Part model, mm, in its own coordinate system. Round coordinates to 2 decimals unless told otherwise and drop trailing zeros. Loops run counter-clockwise (first coordinate to the right, second up) from the corner with the lowest first, then second, coordinate; pieces in that order, holes last.
from build123d import *

# Parameters (mm, degrees)
SKETCH1_R                = 6
BOSS_EXTRUDE1_DEPTH      = 254
BOSS_EXTRUDE1_DEPTH_BACK = 56
CUT_EXTRUDE3_START       = -56
SKETCH2_W                = 4
SKETCH2_H                = 5
CUT_EXTRUDE3_DEPTH       = 20
CUT_EXTRUDE3_DEPTH_BACK  = 0.0001
CUT_EXTRUDE4_START       = 254
SKETCH2_2_W              = 4
SKETCH2_2_H              = 5
CUT_EXTRUDE4_DEPTH       = 50
CUT_EXTRUDE6_START       = -56
SKETCH3_W                = 4
SKETCH3_H                = 10
CUT_EXTRUDE6_DEPTH       = 6


with BuildPart() as part:
    # Sketch1 → Boss-Extrude1 (new body, two sides)
    with BuildSketch(Plane(origin=(0, 0, 0), x_dir=(1, 0, 0), z_dir=(0, 1, 0))) as boss_extrude1_sk:
        Circle(SKETCH1_R)
    extrude(amount=BOSS_EXTRUDE1_DEPTH)
    extrude(boss_extrude1_sk.sketch, amount=-BOSS_EXTRUDE1_DEPTH_BACK)

    # Sketch2 → Cut-Extrude3 (cut, two sides)
    with BuildSketch(Plane(origin=(0, 0, 0), x_dir=(1, 0, 0), z_dir=(0, 1, 0)).offset(CUT_EXTRUDE3_START)) as cut_extrude3_sk:
        with Locations((0, -6)):
            Rectangle(SKETCH2_W, SKETCH2_H)
    extrude(amount=CUT_EXTRUDE3_DEPTH, mode=Mode.SUBTRACT)
    extrude(cut_extrude3_sk.sketch, amount=-CUT_EXTRUDE3_DEPTH_BACK, mode=Mode.SUBTRACT)

    # Sketch2<2> → Cut-Extrude4 (cut)
    with BuildSketch(Plane(origin=(0, 0, 0), x_dir=(1, 0, 0), z_dir=(0, 1, 0)).offset(CUT_EXTRUDE4_START)):
        with Locations((0, -6)):
            Rectangle(SKETCH2_2_W, SKETCH2_2_H)
    extrude(amount=-CUT_EXTRUDE4_DEPTH, mode=Mode.SUBTRACT)

    # Sketch3 → Cut-Extrude6 (cut)
    with BuildSketch(Plane(origin=(0, 0, 0), x_dir=(1, 0, 0), z_dir=(0, 1, 0)).offset(CUT_EXTRUDE6_START)):
        with Locations((0, -6)):
            Rectangle(SKETCH3_W, SKETCH3_H)
    extrude(amount=CUT_EXTRUDE6_DEPTH, mode=Mode.SUBTRACT)


solid = part.part
1) Slice it at A-A, the plane x = 0. Give the cut face in (y, z), then the cut area to 3 significant figures.
Values:
outline: (-56, -6) - (254, -6) - (254, 3.5) - (204, 3.5) - (204, 6) - (-36, 6) - (-36, 3.5) - (-50, 3.5) - (-50, 1) - (-56, 1) - close
area: 3,530 mm2
2) Slice it at B-B, the plane y = 12.5. Give the cut face in (x, z).
Values:
outline: circle Ø12 at (0, 0)
3) Slice it at C-C, the plane z = -2. Give the cut face in (x, y), then the cut area to 3 significant figures.
Values:
outline: (-5.66, -56) - (5.66, -56) - (5.66, 254) - (-5.66, 254) - close
area: 3,510 mm2
4) Wall check: line 1 along X through (y, z) = (216.5, -0.75); line 2 along Y through (x, z) = (1.5, 2.5); line 3 along Z through (x, y) = (-0.75, 234). Give the ranges that are in metal, low to high.
Values:
line 1: x = -5.95 to 5.95
line 2: y = -50 to 254
line 3: z = -5.95 to 3.5
5) Drop flat-ended pins along their axis: pin 1 Ø2 at (y, z) = (132, -2) entering from +X; pin 2 Ø5 at (y, z) = (-43, 3) entering from -X; pin 3 Ø1.2 at (x, y) = (0.5, 235) entering from +Z; pin 4 Ø3 at (x, z) = (-1, 5) entering from +Y. Give the stop position or say it passes through.
Values:
pin 1: stops at x = 5.92
pin 2: stops at x = -5.98
pin 3: stops at z = 3.5
pin 4: stops at y = 254
